Work out the finished part from the listing and answer in its coordinate system (mm). A direction names the side the tool comes from. Give positions to 0.01 mm unless a question says otherwise; leave off trailing zeros. Order: outer loops, then holes, each group sorted by start corner. A loop starts at its lowest first (then second) coordinate and runs counter-clockwise, first axis right, second up.
```python
from build123d import *

# Parameters (mm, degrees)
EXTRUDE_1_DEPTH     = 10
SKETCH_2_W          = 20
SKETCH_2_H          = 20
SKETCH_2_R          = 1.05
CUT_EXTRUDE_2_DEPTH = 8
SKETCH_2_3_R        = 1.05
CUT_EXTRUDE_3_DEPTH = 235.520787991


with BuildPart() as part:
    # Sketch 1 → Extrude 1 (new body)
    with BuildSketch(Plane(origin=(0, 0, 0), x_dir=(1, 0, 0), z_dir=(0, 1, 0))):
        Polygon((-150, -120), (-80, -120), (-80, -180), (-20, -180), (-20, -120), (150, -120), (150, 120), (-150, 120), align=None)
    extrude(amount=EXTRUDE_1_DEPTH)

    # Sketch 2 → Cut-Extrude 2 (cut)
    with BuildSketch(Plane.XZ):
        with Locations((-50, 140)):
            Rectangle(SKETCH_2_W, SKETCH_2_H)
        with Locations(Location((-58, 148, 0), (0, 0, 270))):
            Circle(SKETCH_2_R, mode=Mode.SUBTRACT)
        with Locations(Location((-58, 132, 0), (0, 0, 270))):
            Circle(SKETCH_2_R, mode=Mode.SUBTRACT)
        with Locations(Location((-42, 148, 0), (0, 0, 270))):
            Circle(SKETCH_2_R, mode=Mode.SUBTRACT)
        with Locations(Location((-42, 132, 0), (0, 0, 270))):
            Circle(SKETCH_2_R, mode=Mode.SUBTRACT)
    extrude(amount=-CUT_EXTRUDE_2_DEPTH, mode=Mode.SUBTRACT)

    # Sketch 2_3 → Cut-Extrude 3 (cut, through all)
    with BuildSketch(Plane.XZ):
        with Locations(Location((-42, 132, 0), (0, 0, 270))):
            Circle(SKETCH_2_3_R)
        with Locations(Location((-58, 132, 0), (0, 0, 270))):
            Circle(SKETCH_2_3_R)
        with Locations(Location((-58, 148, 0), (0, 0, 270))):
            Circle(SKETCH_2_3_R)
        with Locations(Location((-42, 148, 0), (0, 0, 270))):
            Circle(SKETCH_2_3_R)
    extrude(amount=-CUT_EXTRUDE_3_DEPTH, mode=Mode.SUBTRACT)


solid = part.part
```
1. Given P1, Ø12, axis at x = -111, z = 42, coming from the -Y side; P2, Ø5, axis at x = -114, y = 3, coming from the +Z side; P3, Ø5, axis at y = 7, z = 152, coming from the +X side; P4, Ø1.9, axis at x = -58, z = 132, coming from the -Y side, each flat-ended and moving along its own axis, determine where each tip first touches the part or whether it passes through.
Findings below:
P1: stops at y = 0
P2: stops at z = 120
P3: stops at x = -20
P4: passes through
2. Which of the six approach directions +Z, -Z, +X, -X, +Y, -Y give full straight-line access (tool end or side, diameter ignored) to faces 4 (the face through (-115, 5, 120)), 5 (the face through (-60, 4, 140)), 6 (the face through (64, 5, 120)), 7 (the face through (-150, 5, -2)), 8 (the face through (-2, 10, -5))?
Findings below:
face 4: +Z, -X, +Y, -Y
face 5: -Y
face 6: +Z, +X, +Y, -Y
face 7: +Z, -Z, -X, +Y, -Y
face 8: +Z, -Z, +X, -X, +Y
3. The part is cut by section A-A (y = 5.5). Write down the section's boundary in (x, z).
Findings below:
outline: (-150, -120) - (150, -120) - (150, 120) - (-20, 120) - (-20, 180) - (-80, 180) - (-80, 120) - (-150, 120) - close; hole (-60, 130) - (-40, 130) - (-40, 150) - (-60, 150) - close
4. The mould has two halves that part along Z. Classify faces 1 (the face through (-50, 4, 130)), 2 (the face through (-20, 5, 150)), 3 (the face through (-50, 5, 180)): pulls with the +Z half, pulls with the -Z half, needs draft (parallel to the pull), parting line crosses it, or undercut.
Findings below:
face 1: undercut
face 2: needs draft
face 3: pulls with the +Z half
5. Straight lines are drawn through the part: probe 1 along X at (y, z) = (9.25, 132); probe 2 along Z at (x, y) = (-49, 2); probe 3 along Z at (x, y) = (125.5, 9). For each, find the intervals that lie inside material, in ascending order.
Findings below:
probe 1: x = -80 to -59.05, -56.95 to -43.05, -40.95 to -20
probe 2: z = -120 to 130, 150 to 180
probe 3: z = -120 to 120
6. The part is cut by section B-B (x = 107). Write down the section's boundary in (y, z), then the cut area to 3 significant figures.
Findings below:
outline: (0, -120) - (10, -120) - (10, 120) - (0, 120) - close
area: 2,400 mm2
